The model under review builds one solid part; all positions refer to its coordinate system, in mm. Give positions to 0.01 mm unless a question says otherwise; leave off trailing zeros. Order: outer loops, then holes, each group sorted by start corner. A loop starts at its lowest first (then second) coordinate and runs counter-clockwise, first axis right, second up. Notation, with made-up numbers: (33, 38) - (75, 38) arc R18 cw to (75, 56) - close; hole circle Ø5 at (19.25, 10.5). An arc over 180 degrees is marked (long way). Put each result on its own line as item: value.
```python
from build123d import *

# Parameters (mm, degrees)
SKETCH1_W               = 520
SKETCH1_H               = 443
SKETCH1_W_2             = 480
SKETCH1_H_2             = 403
BOSS_EXTRUDE2_DEPTH     = 32
SKETCH2_R               = 2.5
CUT_EXTRUDE1_DEPTH      = 610
SKETCH3_R               = 3
CUT_EXTRUDE2_DEPTH      = 641
CUT_EXTRUDE2_DEPTH_BACK = 105


with BuildPart() as part:
    # Sketch1 → Boss-Extrude2 (new body)
    with BuildSketch(Plane(origin=(0, 0, 0), x_dir=(0, 0, -1), z_dir=(1, 0, 0))):
        Rectangle(SKETCH1_W, SKETCH1_H)
        Rectangle(SKETCH1_W_2, SKETCH1_H_2, mode=Mode.SUBTRACT)
    extrude(amount=BOSS_EXTRUDE2_DEPTH)

    # Sketch2 → Cut-Extrude1 (cut)
    with BuildSketch(Plane.XY.offset(260)):
        with Locations((16, -171.5)):
            Circle(SKETCH2_R)
        with Locations((16, -136.5)):
            Circle(SKETCH2_R)
        with Locations((16, -101.5)):
            Circle(SKETCH2_R)
    extrude(amount=-CUT_EXTRUDE1_DEPTH, mode=Mode.SUBTRACT)

    # Sketch3 → Cut-Extrude2 (cut, two sides)
    with BuildSketch(Plane(origin=(0, 0, 240), x_dir=(-1, 0, 0), z_dir=(0, 0, -1))) as cut_extrude2_sk:
        with Locations((-16, 146.5)):
            Circle(SKETCH3_R)
        with Locations((-16, 93.5)):
            Circle(SKETCH3_R)
    extrude(amount=CUT_EXTRUDE2_DEPTH, mode=Mode.SUBTRACT)
    extrude(cut_extrude2_sk.sketch, amount=-CUT_EXTRUDE2_DEPTH_BACK, mode=Mode.SUBTRACT)


solid = part.part
```
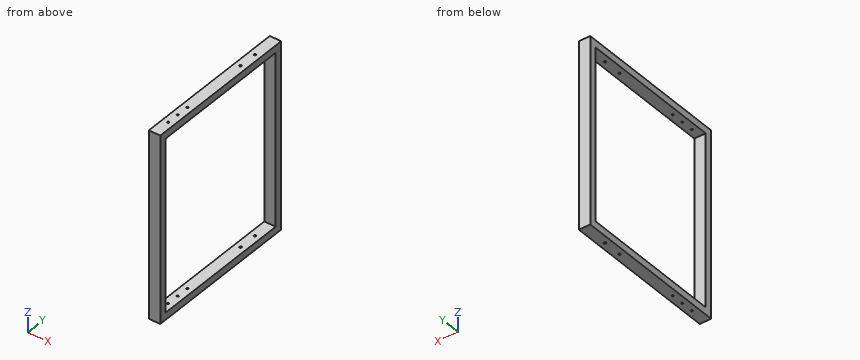
(1) Clearance check with a flat-ended pin moving along its axis: pin 1 Ø4 at (x, y) = (16, -136.5) entering from -Z. State where the tip first meets the part, or that it passes through.
The answers:
pin 1: through
(2) Wall thickness on L1, parallel to Y at x = 16, z = -247.5; L2, parallel to Y at x = 20, z = -84; L3, parallel to Z at x = 8.5, y = -69.5: over which ranges is each line inside the solid? List them lowest first.
The answers:
L1: -221.5 to -174, -169 to -139, -134 to -104, -99 to 90.5, 96.5 to 143.5, 149.5 to 221.5
L2: -221.5 to -201.5, 201.5 to 221.5
L3: -260 to -240, 240 to 260
(3) Take a section at A-A, the plane x = 6. Write out the cut boundary in (y, z).
The answers:
outline: (-221.5, -260) - (221.5, -260) - (221.5, 260) - (-221.5, 260) - close; hole (-201.5, -240) - (201.5, -240) - (201.5, 240) - (-201.5, 240) - close
(4) Take a section at C-C, the plane y = 164.5. Write out the cut boundary in (x, z), then the cut area to 3 significant figures.
The answers:
outline: (0, -260) - (32, -260) - (32, -240) - (0, -240) - close; (0, 240) - (32, 240) - (32, 260) - (0, 260) - close
area: 1,280 mm^2
(5) Take a section at B-B, the plane z = -173.5. Write out the cut boundary in (x, y), then the cut area to 3 significant figures.
The answers:
outline: (0, -221.5) - (32, -221.5) - (32, -201.5) - (0, -201.5) - close; (0, 201.5) - (32, 201.5) - (32, 221.5) - (0, 221.5) - close
area: 1,280 mm^2
